from build123d import *

# Parameters (mm, degrees)
SKETCH1_W           = 133.5
SKETCH1_H           = 70
SKETCH1_R           = 3.05
SKETCH1_R_2         = 2.6
SKETCH1_W_2         = 5
SKETCH1_H_2         = 10
BOSS_EXTRUDE1_DEPTH = 5
FILLET1_R           = 1


with BuildPart() as part:
    # Sketch1 → Boss-Extrude1 (new body)
    with BuildSketch(Plane.XY):
        Rectangle(SKETCH1_W, SKETCH1_H)
        with Locations((25, 22.3)):
            Circle(SKETCH1_R, mode=Mode.SUBTRACT)
        with Locations(Location((-25, 22.3, 0), (0, 0, 180))):
            Circle(SKETCH1_R, mode=Mode.SUBTRACT)
        with Locations((-59.75, -12.5)):
            Circle(SKETCH1_R_2, mode=Mode.SUBTRACT)
        with Locations(Location((59.75, -12.5, 0), (0, 0, 180))):
            Circle(SKETCH1_R_2, mode=Mode.SUBTRACT)
        with Locations(Location((-59.75, 12.5, 0), (0, 0, 180))):
            Circle(SKETCH1_R_2, mode=Mode.SUBTRACT)
        with Locations((59.75, 12.5)):
            Circle(SKETCH1_R_2, mode=Mode.SUBTRACT)
        with Locations((25, -27.7)):
            Circle(SKETCH1_R, mode=Mode.SUBTRACT)
        with Locations(Location((-25, -27.7, 0), (0, 0, 180))):
            Circle(SKETCH1_R, mode=Mode.SUBTRACT)
        with Locations((-59.75, -25)):
            Rectangle(SKETCH1_W_2, SKETCH1_H_2, mode=Mode.SUBTRACT)
        with Locations((59.75, -25)):
            Rectangle(SKETCH1_W_2, SKETCH1_H_2, mode=Mode.SUBTRACT)
        with Locations((-59.75, 0)):
            Rectangle(SKETCH1_W_2, SKETCH1_H_2, mode=Mode.SUBTRACT)
        with Locations((59.75, 0)):
            Rectangle(SKETCH1_W_2, SKETCH1_H_2, mode=Mode.SUBTRACT)
        with Locations((-59.75, 25)):
            Rectangle(SKETCH1_W_2, SKETCH1_H_2, mode=Mode.SUBTRACT)
        with Locations((59.75, 25)):
            Rectangle(SKETCH1_W_2, SKETCH1_H_2, mode=Mode.SUBTRACT)
    extrude(amount=BOSS_EXTRUDE1_DEPTH)

    # Fillet1
    fillet1_edges = [part.edges().sort_by_distance(p)[0] for p in [
        (66.75, -35, 2.5),
        (-66.75, -35, 2.5),
        (-66.75, 35, 2.5),
        (66.75, 35, 2.5),
    ]]
    fillet(fillet1_edges, radius=FILLET1_R)


solid = part.part
Input: part model. Units: mm. Frame: model coordinates. Give positions to 0.01 mm unless a question says otherwise; leave off trailing zeros. Loops run counter-clockwise (first coordinate to the right, second up) from the corner with the lowest first, then second, coordinate; pieces in that order, holes last. Notation, with made-up numbers: (48.5, -38.5) - (107.5, -38.5) arc R22 ccw to (107.5, -19.5) - close; hole circle Ø7 at (-29, 70.25). An arc over 180 degrees is marked (long way). Use CSV: the item, a comma, the result in double quotes. Start each with the question number.
Item 1: Section B-B on y = 12.5. Return loops of the section in (x, z).
Item 2: Line query: line 1 (X direction, y = 4, z = 4.75); line 2 (Y direction, x = -25, z = 2); line 3 (Y direction, x = 59.75, z = 2.6). Output: solid intervals per line, ascending.
Item 3: Section D-D on x = 59.75. Return loops of the section in (y, z), then the cut area to 3 significant figures.
Item 4: Contact query for a flat-ended pin moving along its axis: P1, Ø3, axis at x = -4, y = 14, coming from the -Z side. Output: stop coordinate, or through.
Item 5: Section C-C on x = 25. Return loops of the section in (y, z), then the cut area to 3 significant figures.
Item 6: Section A-A on y = 22.3. Return loops of the section in (x, z).
Item 7: Mould query, pull axis Y, two halves, no side actions, for faces 1 (the flat face through (-1, -35, 2)), 2 (the flat face through (60, 20, 2)), 3 (the flat face through (-1, 35, 2)). Classes: pulls with the +Y half, pulls with the -Y half, needs draft (parallel to the pull), parting line crosses it, or undercut.
Ans:
1,outline,"(-66.75, 0) - (-62.35, 0) - (-62.35, 5) - (-66.75, 5) - close; (-57.15, 0) - (57.15, 0) - (57.15, 5) - (-57.15, 5) - close; (62.35, 0) - (66.75, 0) - (66.75, 5) - (62.35, 5) - close"
2,line 1,"x = -66.75 to -62.25, -57.25 to 57.25, 62.25 to 66.75"
2,line 2,"y = -35 to -30.75, -24.65 to 19.25, 25.35 to 35"
2,line 3,"y = -35 to -30, -20 to -15.1, -9.9 to -5, 5 to 9.9, 15.1 to 20, 30 to 35"
3,outline,"(-35, 0) - (-30, 0) - (-30, 5) - (-35, 5) - close; (-20, 0) - (-15.1, 0) - (-15.1, 5) - (-20, 5) - close; (-9.9, 0) - (-5, 0) - (-5, 5) - (-9.9, 5) - close; (5, 0) - (9.9, 0) - (9.9, 5) - (5, 5) - close; (15.1, 0) - (20, 0) - (20, 5) - (15.1, 5) - close; (30, 0) - (35, 0) - (35, 5) - (30, 5) - close"
3,area,"148 mm2"
4,P1,"stops at z = 0"
5,outline,"(-35, 0) - (-30.75, 0) - (-30.75, 5) - (-35, 5) - close; (-24.65, 0) - (19.25, 0) - (19.25, 5) - (-24.65, 5) - close; (25.35, 0) - (35, 0) - (35, 5) - (25.35, 5) - close"
5,area,"289 mm2"
6,outline,"(-66.75, 0) - (-62.25, 0) - (-62.25, 5) - (-66.75, 5) - close; (-57.25, 0) - (-28.05, 0) - (-28.05, 5) - (-57.25, 5) - close; (-21.95, 0) - (21.95, 0) - (21.95, 5) - (-21.95, 5) - close; (28.05, 0) - (57.25, 0) - (57.25, 5) - (28.05, 5) - close; (62.25, 0) - (66.75, 0) - (66.75, 5) - (62.25, 5) - close"
7,face 1,"pulls with the -Y half"
7,face 2,"undercut"
7,face 3,"pulls with the +Y half"
